Input: part model. Units: mm. Frame: model coordinates. Coordinates: 2 decimals unless noted, no trailing zeros. Loops run counter-clockwise (first coordinate to the right, second up) from the corner with the lowest first, then second, coordinate; pieces in that order, holes last.
```python
from build123d import *

# Parameters (mm, degrees)
F5_R     = 3.175
F6_DEPTH = 50.8


# Not quite as in the source:
# - a length typed as a fraction of an inch, garbled in the dataset ("3 / 203.2 mm" for 3/8 in), is restored


with BuildPart() as f2:
    # F0 (on Front) → F2 (revolve)
    with BuildSketch(Plane.XZ):
        with BuildLine():
            Line((0, -15.875), (0, 15.875))
            ThreePointArc((0, 15.875), (-15.875, 0), (0, -15.875))
        make_face()
    revolve(axis=Axis((0, 0, 0), (0, 0, 1)))


with BuildPart() as f6:
    # F5 (on offset) → F6 (new body)
    with BuildSketch(Plane.XY.offset(5.715)):
        Circle(F5_R)
    extrude(amount=F6_DEPTH)


with BuildPart() as f2_1:
    add(f2.part)

    # F7: cut F6
    add(f6.part, mode=Mode.SUBTRACT)


solid = f2_1.part
```
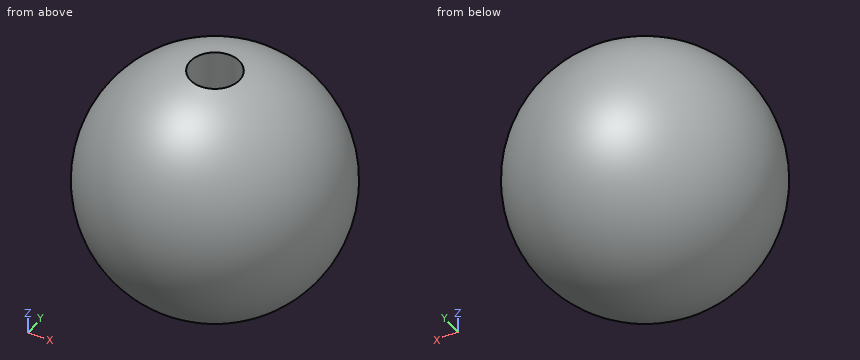
Item 1: Section query A-A (x = 0). Output: boundary loops of the cut face in (y, z) (3 decimals), then the cut area to 3 significant figures.
Result:
outline: (-3.175, 5.715) - (-3.175, 15.554) arc R15.875 ccw (long way) to (3.175, 15.554) - (3.175, 5.715) - close
area: 728 mm2
Item 2: Section query C-C (z = -8.5). Output: boundary loops of the cut face in (x, y), then the cut area to 3 significant figures.
Result:
outline: circle Ø26.82 at (0, 0)
area: 565 mm2
Item 3: Contact query for flat-ended pins moving along their axis: P1, Ø8.5, axis at x = 0, y = 0, coming from the +Z side; P2, Ø1.5, axis at y = -7.5, z = 1.5, coming from the +X side; P3, Ø3, axis at x = 8, y = -2, coming from the -Z side; P4, Ø1, axis at y = -8.5, z = 7.5, coming from the -X side. Output: stop coordinate, or through.
Result:
P1: stops at z = 15.55
P2: stops at x = 14.3
P3: stops at z = -14.37
P4: stops at x = -11.6
Item 4: Line query: L1, parallel to X at y = 1.5, z = 12.5; L2, parallel to Y at x = 0, z = 11.5 (3 decimals); L3, parallel to Y at x = 0, z = 8 (3 decimals). Output: solid intervals per line, ascending.
Result:
L1: x = -9.67 to -2.8, 2.8 to 9.67
L2: y = -10.944 to -3.175, 3.175 to 10.944
L3: y = -13.712 to -3.175, 3.175 to 13.712
Item 5: Section query D-D (z = 7). Output: boundary loops of the cut face in (x, y) (3 decimals).
Result:
outline: circle Ø28.497 at (0, 0); hole circle Ø6.35 at (0, 0)
